Read the model definition and answer for the solid it produces. Units are mm, in the model's axes. A direction names the side the tool comes from. Coordinates: 2 decimals unless noted, no trailing zeros. Loops run counter-clockwise (first coordinate to the right, second up) from the corner with the lowest first, then second, coordinate; pieces in that order, holes last. Notation, with made-up numbers: M 70,37 L 88,37 A18 cw 88,46 Z; hole C 47,36 d11. An arc over 180 degrees is marked long. One line per item, written item: value. Start each with the question number.
1. Determine the mould class of faces 4 (the face through (75.82, 1.48, -51)), 5 (the face through (98, 1, 32.5)), 6 (the face through (112, 1, 37)) for opening direction Z: +Z half, -Z half, draft (parallel to the pull), parting line (faces both ways), or undercut.
2. Consider probe 1 along X at (y, z) = (2.6, -23); probe 2 along Z at (x, y) = (100.5, 0.15); probe 3 along Z at (x, y) = (150, 2.9). Determine where each line is inside the solid, lowest interval first.
3. Flat-ended cylindrical pins translate along their axes: pin 1 (1.5 mm diameter, centred on x = 127.5, y = 1.5, fed in from +Z); pin 2 (2 mm diameter, centred on x = 83.85, z = 23, fed in from +Y) (3 decimals); pin 3 (1.5 mm diameter, centred on x = 99.5, y = 1, fed in from +Z); pin 4 (0.9 mm diameter, centred on y = 1, z = -27.5, fed in from +X). Find the tip coordinate at first contact, or state that the pin passes through.
4. The part is cut by section C-C (y = 1.05). State how many separate pieces and enclosed holes the cut face has, then the cut area to 3 significant figures.
5. For faces 1 (the face through (165.03, 1.48, 38.21)), 2 (the face through (126, 1, -28.5)), 3 (the face through (58.667, 1.479, -34.209)), determine the directions among +Z, -Z, +X, -X, +Y, -Y from which every point of the face is accessible in a straight line to the end or side of a thin tool.
6. The part is cut by section D-D (x = 136). Write down the section's boundary in (y, z).
7. The part is cut by section A-A (z = 13.5). Write down the section's boundary in (x, y), then the cut area to 3 significant figures.
8. The part is cut by section B-B (z = -17). Write down the section's boundary in (x, y).
```python
from build123d import *

# Parameters (mm, degrees)
ESBO_O1_R                = 1.5
ESBO_O1_R_2              = 1.25
ESBO_O1_R_3              = 2.5
ESBO_O1_W                = 8
ESBO_O1_H                = 3
RESSALTO_EXTRUS_O1_DEPTH = 3


with BuildPart() as part:
    # Esboço1 → Ressalto-extrusão1 (new body)
    with BuildSketch(Plane(origin=(0, 0, 0), x_dir=(1, 0, 0), z_dir=(0, 1, 0))):
        with BuildLine():
            Line((52.381074728, 40.494515949), (65.131240604, 27.744350072))
            ThreePointArc((65.131240604, 27.744350072), (73.802150657, 14.76741612), (76.846969357, -0.539921175))
            Line((76.846969357, -0.539921175), (76.846969357, -3.460078825))
            ThreePointArc((76.846969357, -3.460078825), (73.802150657, -18.76741612), (65.131240604, -31.744350072))
            Line((65.131240604, -31.744350072), (52.381074728, -44.494515949))
            ThreePointArc((52.381074728, -44.494515949), (55.208930541, -58.638038816), (69.352453408, -61.465894629))
            Line((69.352453408, -61.465894629), (82.102619284, -48.715728753))
            ThreePointArc((82.102619284, -48.715728753), (95.079553237, -40.0448187), (110.386890532, -37))
            Line((110.386890532, -37), (113.308680045, -37))
            ThreePointArc((113.308680045, -37), (128.61601734, -40.0448187), (141.592951292, -48.715728753))
            Line((141.592951292, -48.715728753), (154.343117169, -61.465894629))
            ThreePointArc((154.343117169, -61.465894629), (168.486640036, -58.638038816), (171.314495849, -44.494515949))
            Line((171.314495849, -44.494515949), (158.564329973, -31.744350072))
            ThreePointArc((158.564329973, -31.744350072), (149.89341992, -18.76741612), (146.84860122, -3.460078825))
            Line((146.84860122, -3.460078825), (146.84860122, -0.539921175))
            ThreePointArc((146.84860122, -0.539921175), (149.89341992, 14.76741612), (158.564329973, 27.744350072))
            Line((158.564329973, 27.744350072), (171.314495849, 40.494515949))
            ThreePointArc((171.314495849, 40.494515949), (168.486640036, 54.638038816), (154.343117169, 57.465894629))
            Line((154.343117169, 57.465894629), (141.592951292, 44.715728753))
            ThreePointArc((141.592951292, 44.715728753), (128.61601734, 36.0448187), (113.308680045, 33))
            Line((113.308680045, 33), (110.386890532, 33))
            ThreePointArc((110.386890532, 33), (95.079553237, 36.0448187), (82.102619284, 44.715728753))
            Line((82.102619284, 44.715728753), (69.352453408, 57.465894629))
            ThreePointArc((69.352453408, 57.465894629), (55.208930541, 54.638038816), (52.381074728, 40.494515949))
        make_face()
        with Locations(Location((111.847785288, 27, 0), (0, 0, 270))):
            Circle(ESBO_O1_R, mode=Mode.SUBTRACT)
        with Locations(Location((111.847785288, -31, 0), (0, 0, 270))):
            Circle(ESBO_O1_R, mode=Mode.SUBTRACT)
        with Locations(Location((60.796461355, 48.909902577, 0), (0, 0, 270))):
            Circle(ESBO_O1_R, mode=Mode.SUBTRACT)
        with Locations(Location((111.847785288, -13.5, 0), (0, 0, 270))):
            Circle(ESBO_O1_R, mode=Mode.SUBTRACT)
        with Locations(Location((124.847785288, -13.5, 0), (0, 0, 270))):
            Circle(ESBO_O1_R, mode=Mode.SUBTRACT)
        with Locations(Location((98.847785288, -13.5, 0), (0, 0, 270))):
            Circle(ESBO_O1_R, mode=Mode.SUBTRACT)
        with Locations(Location((98.847785288, 9.5, 0), (0, 0, 270))):
            Circle(ESBO_O1_R, mode=Mode.SUBTRACT)
        with Locations(Location((124.847785288, 9.5, 0), (0, 0, 270))):
            Circle(ESBO_O1_R, mode=Mode.SUBTRACT)
        with Locations(Location((111.847785288, 9.5, 0), (0, 0, 270))):
            Circle(ESBO_O1_R, mode=Mode.SUBTRACT)
        with Locations(Location((83.847785288, -4, 0), (0, 0, 270))):
            Circle(ESBO_O1_R_2, mode=Mode.SUBTRACT)
        with Locations(Location((139.847785288, -4, 0), (0, 0, 270))):
            Circle(ESBO_O1_R_2, mode=Mode.SUBTRACT)
        with Locations(Location((60.796461355, -52.909902577, 0), (0, 0, 270))):
            Circle(ESBO_O1_R, mode=Mode.SUBTRACT)
        with Locations(Location((139.847785288, -23, 0), (0, 0, 270))):
            Circle(ESBO_O1_R_2, mode=Mode.SUBTRACT)
        with Locations(Location((83.847785288, -23, 0), (0, 0, 270))):
            Circle(ESBO_O1_R_2, mode=Mode.SUBTRACT)
        with Locations(Location((112.847785288, 17, 0), (0, 0, 270))):
            Circle(ESBO_O1_R, mode=Mode.SUBTRACT)
        with Locations(Location((162.899109221, -52.909902577, 0), (0, 0, 270))):
            Circle(ESBO_O1_R, mode=Mode.SUBTRACT)
        with Locations(Location((162.899109221, 48.909902577, 0), (0, 0, 270))):
            Circle(ESBO_O1_R, mode=Mode.SUBTRACT)
        with Locations(Location((142.847785288, 1, 0), (0, 0, 270))):
            Circle(ESBO_O1_R, mode=Mode.SUBTRACT)
        with Locations(Location((80.903069614, 23.804170545, 0), (0, 0, 270))):
            Circle(ESBO_O1_R_3, mode=Mode.SUBTRACT)
        with Locations(Location((87.129249486, 23.804170545, 0), (0, 0, 270))):
            Circle(ESBO_O1_R_3, mode=Mode.SUBTRACT)
        with Locations((125.847785288, -31)):
            Rectangle(ESBO_O1_W, ESBO_O1_H, mode=Mode.SUBTRACT)
        Polygon((149.102405747, 37.250212448), (151.223726091, 39.371532792), (153.345046434, 37.250212448), (151.223726091, 35.128892104), align=None, mode=Mode.SUBTRACT)
        Polygon((154.052153215, 42.199959916), (156.173473559, 44.32128026), (158.294793903, 42.199959916), (156.173473559, 40.078639573), align=None, mode=Mode.SUBTRACT)
        with Locations((97.847785288, -31)):
            Rectangle(ESBO_O1_W, ESBO_O1_H, mode=Mode.SUBTRACT)
        with Locations((97.847785288, 27)):
            Rectangle(ESBO_O1_W, ESBO_O1_H, mode=Mode.SUBTRACT)
        with Locations((125.847785288, 27)):
            Rectangle(ESBO_O1_W, ESBO_O1_H, mode=Mode.SUBTRACT)
        Polygon((67.522097018, 44.32128026), (65.400776674, 42.199959916), (67.522097018, 40.078639573), (69.643417361, 42.199959916), align=None, mode=Mode.SUBTRACT)
        Polygon((72.471844486, 39.371532792), (70.350524142, 37.250212448), (72.471844486, 35.128892104), (74.593164829, 37.250212448), align=None, mode=Mode.SUBTRACT)
        Polygon((67.522097018, -44.078639573), (65.400776674, -46.199959916), (67.522097018, -48.32128026), (69.643417361, -46.199959916), align=None, mode=Mode.SUBTRACT)
        Polygon((74.593164829, -41.250212448), (72.471844486, -43.371532792), (70.350524142, -41.250212448), (72.471844486, -39.128892104), align=None, mode=Mode.SUBTRACT)
        Polygon((156.173473559, -48.32128026), (158.294793903, -46.199959916), (156.173473559, -44.078639573), (154.052153215, -46.199959916), align=None, mode=Mode.SUBTRACT)
        Polygon((151.223726091, -43.371532792), (153.345046434, -41.250212448), (151.223726091, -39.128892104), (149.102405747, -41.250212448), align=None, mode=Mode.SUBTRACT)
    extrude(amount=RESSALTO_EXTRUS_O1_DEPTH)


solid = part.part
```
Answer block:
1. face 4: -Z half
1. face 5: undercut
1. face 6: +Z half
2. probe 1: x = 69.19 to 78.54, 83.27 to 84.76, 89.5 to 154.51
2. probe 2: z = -34.24 to -28.5, -25.5 to 29.5, 32.5 to 38.24
2. probe 3: z = -53.12 to -38.15, -36.35 to -15.02, 19.02 to 40.35, 42.15 to 57.12
3. pin 1: stops at z = 39.9
3. pin 2: passes through
3. pin 3: stops at z = 38.73
3. pin 4: stops at x = 158.77
4. separate pieces: 1
4. enclosed holes: 32
4. area: 8,150 mm2
5. face 1: +X, +Y, -Y
5. face 2: +Y, -Y
5. face 3: -X, +Y, -Y
6. outline: M 0,-40.06 L 3,-40.06 L 3,44.06 L 0,44.06 Z
7. outline: M 75.57,0 L 97.35,0 L 97.35,3 L 75.57,3 Z; M 100.35,0 L 110.35,0 L 110.35,3 L 100.35,3 Z; M 113.35,0 L 123.35,0 L 123.35,3 L 113.35,3 Z; M 126.35,0 L 148.13,0 L 148.13,3 L 126.35,3 Z
7. area: 191 mm2
8. outline: M 72.8,0 L 111.35,0 L 111.35,3 L 72.8,3 Z; M 114.35,0 L 150.9,0 L 150.9,3 L 114.35,3 Z
